```python
from build123d import *

# Parameters (mm, degrees)
F0_R     = 196.85
F1_DEPTH = 38.1
F0_R_2   = 171.45
F2_DEPTH = 19.05
F3_R     = 9.525


with BuildPart() as f1:
    # F0 (on Top) → F1 (new body)
    with BuildSketch(Plane.XY):
        with BuildLine():
            Line((0, 355.6), (0, 0))
            Line((0, 0), (1016, 0))
            Line((1016, 0), (1016, 355.6))
            ThreePointArc((1016, 355.6), (986.242049, 427.442049), (914.4, 457.2))
            Line((914.4, 457.2), (101.6, 457.2))
            ThreePointArc((101.6, 457.2), (29.757951, 427.442049), (0, 355.6))
        make_face()
        with Locations((266.7, 215.9)):
            Circle(F0_R, mode=Mode.SUBTRACT)
        with Locations((749.3, 215.9)):
            Circle(F0_R, mode=Mode.SUBTRACT)
    extrude(amount=F1_DEPTH)

    # F0 (on Top) → F2 (join)
    with BuildSketch(Plane.XY):
        with Locations((266.7, 215.9)):
            Circle(F0_R)
        with Locations((266.7, 215.9)):
            Circle(F0_R_2, mode=Mode.SUBTRACT)
        with Locations((749.3, 215.9)):
            Circle(F0_R)
        with Locations((749.3, 215.9)):
            Circle(F0_R_2, mode=Mode.SUBTRACT)
    extrude(amount=F2_DEPTH)

    # F3
    f3_edges = [f1.edges().sort_by_distance(p)[0] for p in [
        (69.85, 215.9, 38.1),
        (552.45, 215.9, 38.1),
    ]]
    fillet(f3_edges, radius=F3_R)


solid = f1.part
```
Design review of the part built by this model. Coordinates are the model's own, in mm. A direction names the side the tool comes from. Coordinates: 2 decimals unless noted, no trailing zeros. Order: outer loops, then holes, each group sorted by start corner. A loop starts at its lowest first (then second) coordinate and runs counter-clockwise, first axis right, second up.
1) Clearance check with flat-ended pins moving along their axes: pin 1 (2 mm diameter, centred on y = 396.5, z = 6.5, fed in from +X); pin 2 (10 mm diameter, centred on x = 893.5, z = 18.5, fed in from -Y). State where each tip first meets the part, or that it passes through.
2) Take a section at C-C, the plane z = 9.5. Give the boundary of the cut face in (x, y), and give its area (3 significant figures).
3) Take a section at B-B, the plane y = 215.9. Give the boundary of the cut face in (x, z) (3 decimals), and give its area (3 significant figures).
4) For faces 1 (the cylindrical face through (30.552, 428.228, 18.783)), 2 (the cylindrical face through (840.13, 41.26, 23.75)), list the 3-axis set-ups (+Z, -Z, +X, -X, +Y, -Y) from which the entire face can be reached by the end or side of a thin tool; tool diameter is ignored.
5) Wall thickness on line 1 along X through (y, z) = (215, 24); line 2 along Y through (x, z) = (749.3, 15); line 3 along X through (y, z) = (122, 4): over which ranges is each line inside the solid? List them lowest first.
6) Take a section at D-D, the plane y = 266. State how many separate pieces and enclosed holes the cut face has, and give its area (3 significant figures).
7) Mouldability with a two-part tool opening along X and no side actions: class faces 3 (the flat face through (501, 232, 38.1)), 4 (the flat face through (1016, 175, 19)), 5 (the cylindrical face through (110.5, 96.1, 23.7)), 6 (the flat face through (207, 377, 19.05)) as +X half, -X half, draft (parallel to the pull), parting line (faces both ways), or undercut.
8) Take a section at A-A, the plane x = 749.3. Give the boundary of the cut face in (y, z) (3 decimals), and give its area (3 significant figures).
Returned:
1. pin 1: stops at x = 1007.84
1. pin 2: stops at y = 0
2. outline: (0, 0) - (1016, 0) - (1016, 355.6) arc R101.6 ccw to (914.4, 457.2) - (101.6, 457.2) arc R101.6 ccw to (0, 355.6) - close; hole circle Ø342.9 at (266.7, 215.9); hole circle Ø342.9 at (749.3, 215.9)
2. area: 275,000 mm2
3. outline: (0, 0) - (95.25, 0) - (95.25, 19.05) - (69.85, 19.05) - (69.85, 28.575) arc R9.525 ccw to (60.325, 38.1) - (0, 38.1) - close; (438.15, 0) - (577.85, 0) - (577.85, 19.05) - (552.45, 19.05) - (552.45, 28.575) arc R9.525 ccw to (542.925, 38.1) - (473.075, 38.1) arc R9.525 ccw to (463.55, 28.575) - (463.55, 19.05) - (438.15, 19.05) - close; (920.75, 0) - (1016, 0) - (1016, 38.1) - (955.675, 38.1) arc R9.525 ccw to (946.15, 28.575) - (946.15, 19.05) - (920.75, 19.05) - close
3. area: 10,600 mm2
4. face 1: +Z, -Z, -X, +Y
4. face 2: +Z
5. line 1: x = 0 to 69.85, 463.55 to 552.45, 946.15 to 1016
5. line 2: y = 0 to 44.45, 387.35 to 457.2
5. line 3: x = 0 to 123.25, 410.15 to 605.85, 892.75 to 1016
6. separate pieces: 3
6. enclosed holes: 0
6. area: 11,600 mm2
7. face 3: draft
7. face 4: +X half
7. face 5: undercut
7. face 6: undercut
8. outline: (0, 0) - (44.45, 0) - (44.45, 19.05) - (19.05, 19.05) - (19.05, 28.575) arc R9.525 ccw to (9.525, 38.1) - (0, 38.1) - close; (387.35, 0) - (457.2, 0) - (457.2, 38.1) - (422.275, 38.1) arc R9.525 ccw to (412.75, 28.575) - (412.75, 19.05) - (387.35, 19.05) - close
8. area: 3,350 mm2
